Source: CAD feature listing. Evaluate the final solid. Frame: model axes, mm. Face numbers are marked on the shaded views. A direction names the side the tool comes from. Coordinates: 2 decimals unless noted, no trailing zeros. Write each loop counter-clockwise with the first axis right and the second up, starting at its lowest first coordinate (ties: lowest second). Pieces come first, ordered by that corner, then holes. Notation, with made-up numbers: (-3.75, 1) - (24.25, 1) arc R9 ccw to (24.25, 13) - close; hole circle Ø8 at (19, 71). An arc over 180 degrees is marked (long way). One line per question, with ' | ' between items.
from build123d import *

# Parameters (mm, degrees)
EXTRUDE_1_DEPTH     = 5
SKETCH_8_OUTSIDE_W  = 22.464
SKETCH_8_OUTSIDE_H  = 20.522
SKETCH_8_OUTSIDE_R  = 6.278684177
CUT_EXTRUDE_1_DEPTH = 1
CUT_EXTRUDE_1_DRAFT = -45
SKETCH_9_R          = 3.825
BOLT_LENGTH_DEPTH   = 60
FILLET_1_R          = 1
CHAMFER_1_SIZE      = 1


with BuildPart() as part:
    # Эскиз6 → Бобышка-Вытянуть1 (new body)
    with BuildSketch(Plane(origin=(0, 0, 0), x_dir=(1, 0, 0), z_dir=(0, 1, 0))):
        Polygon((7.25, 0), (3.625, 6.278684177), (-3.625, 6.278684177), (-7.25, 0), (-3.625, -6.278684177), (3.625, -6.278684177), align=None)
    extrude(amount=EXTRUDE_1_DEPTH)


with BuildPart() as cut_extrude_1_tool:
    # Эскиз8 outside → Вырез-Вытянуть1 (with draft: the straight prism first)
    with BuildSketch(Plane(origin=(0, 5, 0), x_dir=(1, 0, 0), z_dir=(0, 1, 0))):
        Rectangle(SKETCH_8_OUTSIDE_W, SKETCH_8_OUTSIDE_H)
        Circle(SKETCH_8_OUTSIDE_R, mode=Mode.SUBTRACT)
    extrude(amount=-CUT_EXTRUDE_1_DEPTH)
    # Вырез-Вытянуть1: the draft: its side faces are tilted about the plane it starts from
    cut_extrude_1_sides = [cut_extrude_1_tool.faces().sort_by_distance(p)[0] for p in [
        (0, 4.5, 10.261),
        (11.232, 4.5, 0),
        (0, 4.5, -10.261),
        (-11.232, 4.5, 0),
        (-6.278684177, 4.5, 0),
    ]]
    draft(cut_extrude_1_sides, Plane(origin=(0, 5, 0), x_dir=(1, 0, 0), z_dir=(0, 1, 0)), CUT_EXTRUDE_1_DRAFT)


with BuildPart() as part_1:
    add(part.part)

    # Вырез-Вытянуть1: cut by cut_extrude_1_tool
    add(cut_extrude_1_tool.part, mode=Mode.SUBTRACT)

    # Эскиз9 → bolt length (add)
    with BuildSketch(Plane.XZ):
        with Locations(Location((0, 0, 0), (0, 0, 90))):  # turned: the seam where the file's is
            Circle(SKETCH_9_R)
    extrude(amount=BOLT_LENGTH_DEPTH)

    # Скругление1
    fillet_1_edges = [part_1.edges().sort_by_distance(p)[0] for p in [
        (0, 0, -3.825),
    ]]
    fillet(fillet_1_edges, radius=FILLET_1_R)

    # Фаска1
    chamfer_1_edges = [part_1.edges().sort_by_distance(p)[0] for p in [
        (0, -60, -3.825),
    ]]
    chamfer(chamfer_1_edges, length=CHAMFER_1_SIZE)


solid = part_1.part
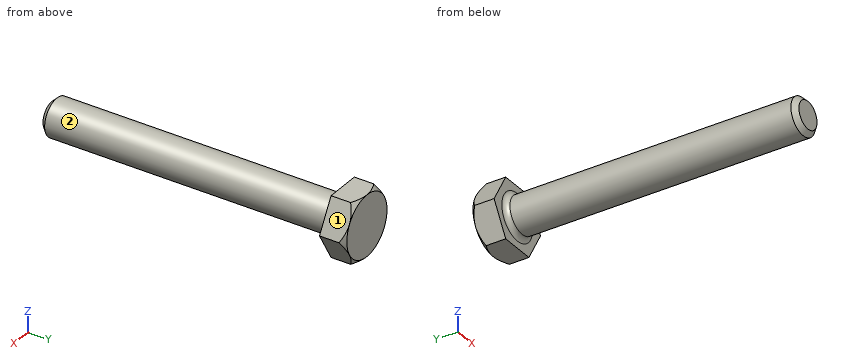
Item 1: Ray query, line 1 along Z through (x, y) = (1.25, -56.5); line 2 along Y through (x, z) = (-3, -4); line 3 along X through (y, z) = (-50, 3.5). Return the intervals inside material, ascending. Write a range as [from, to].
Check sheet entries:
line 1: [-3.61, 3.61] | line 2: [0, 5] | line 3: [-1.54, 1.54]
Item 2: Access query for the marked faces 1 and 2. Directions: +Z, -Z, +X, -X, +Y, -Y. A direction counts if a zero-diameter tool reaches every point of the face in a straight line with its end or side. Return the directions, or none.
Check sheet entries:
face 1: +Z, +X, +Y, -Y | face 2: -Y
Item 3: Cut plane A-A on y = -9.5. Return loops of the section in (x, z) (3 decimals).
Check sheet entries:
outline: circle Ø7.65 at (0, 0)
Item 4: Pin query (flat end, axial travel): pin 1 Ø3 at (x, y) = (-2, -29.5) entering from -Z; pin 2 Ø3 at (y, z) = (-44, -2) entering from +X; pin 3 Ø1.5 at (y, z) = (-7.5, -2.5) entering from +X. Return the tip coordinate at first contact, or that it passes through.
Check sheet entries:
pin 1: z = -3.79 | pin 2: x = 3.79 | pin 3: x = 3.4
